```python
from build123d import *

# Parameters (mm, degrees)
F0_R     = 12.7
F1_DEPTH = 25.4
F2_R     = 12.7
F3_DEPTH = 50.8
F4_R     = 12.7


with BuildPart() as f1:
    # F0 (on Front) → F1 (new body)
    with BuildSketch(Plane.XZ):
        with BuildLine():
            Line((60.317927, -4.766353), (-27.044199, 54.367976))
            ThreePointArc((-27.044199, 54.367976), (-53.188332, 55.770247), (-66.682073, 33.333647))
            Line((-66.682073, 33.333647), (-66.682073, -17.466353))
            Line((-66.682073, -17.466353), (60.317927, -17.466353))
            Line((60.317927, -17.466353), (60.317927, -4.766353))
        make_face()
        with Locations((-41.282073, 33.333647)):
            Circle(F0_R, mode=Mode.SUBTRACT)
    extrude(amount=F1_DEPTH)

    # F2 (on Front) → F3 (join)
    with BuildSketch(Plane.XZ):
        with BuildLine():
            Line((-15.862083, -4.67199), (-15.862083, 33.193771))
            ThreePointArc((-15.862083, 33.193771), (-41.262083, 58.593771), (-66.662083, 33.193771))
            ThreePointArc((-66.662083, 33.193771), (-66.662036, 33.145056), (-66.661896, 33.096341))
            Line((-66.661896, 33.096341), (-66.58946, -4.67199))
            Line((-66.58946, -4.67199), (-66.58946, -17.566571))
            Line((-66.58946, -17.566571), (60.406737, -17.566571))
            Line((60.406737, -17.566571), (60.406737, -4.67199))
            Line((60.406737, -4.67199), (-15.862083, -4.67199))
        make_face()
        with Locations((-41.262083, 33.193771)):
            Circle(F2_R, mode=Mode.SUBTRACT)
    extrude(amount=F3_DEPTH)

    # F4
    f4_edges = [f1.edges().sort_by_distance(p)[0] for p in [
        (60.406737, -50.8, -11.11928),
    ]]
    fillet(f4_edges, radius=F4_R)


solid = f1.part
```
Geometry: final body of the model. Coordinates: model frame, mm. A direction names the side the tool comes from. Coordinates: 2 decimals unless noted, no trailing zeros. Loops run counter-clockwise (first coordinate to the right, second up) from the corner with the lowest first, then second, coordinate; pieces in that order, holes last. Notation, with made-up numbers: M 41,30.25 L 98,30.25 A21 ccw 98,45.25 Z; hole C -18,49.5 d11. An arc over 180 degrees is marked long. Put each result on its own line as item: value.
(1) Material intervals for probe 1 along X at (y, z) = (-31, -5); probe 2 along X at (y, z) = (-6, 39); probe 3 along Z at (x, y) = (-27, -17), sorted ascending.
Answer sheet:
probe 1: x = -66.59 to 60.41
probe 2: x = -66.04 to -52.56, -29.97 to -4.34
probe 3: z = -17.57 to 54.34
(2) Cut plane A-A on y = -34. Return the cut outline in (x, z).
Answer sheet:
outline: M -66.66,33.1 L -66.59,-4.67 L -66.59,-17.57 L 60.41,-17.57 L 60.41,-4.67 L -15.86,-4.67 L -15.86,33.19 A25.4 ccw -66.66,33.19 A25.52 ccw Z; hole C -41.26,33.19 d25.4
(3) Cut plane D-D on z = 9.5. Return the cut outline in (x, y).
Answer sheet:
outline: M -66.68,-25.4 L -66.62,-25.4 L -66.62,-50.8 L -15.86,-50.8 L -15.86,-25.4 L 39.24,-25.4 L 39.24,0 L -66.68,0 Z
(4) Draft query along X for faces 1 (the face through (-39.761, -12.522, 20.725)), 2 (the face through (-52.847, -12.522, 55.948)), 3 (the face through (-15.862, -38, 14)). Return one class per face: pulls with the +X half, pulls with the -X half, needs draft (parallel to the pull), parting line crosses it, or undercut.
Answer sheet:
face 1: undercut
face 2: parting line crosses it
face 3: pulls with the +X half
(5) Cut plane C-C on z = 40.5. Return the cut outline in (x, y).
Answer sheet:
outline: M -65.65,-25.4 L -65.59,-25.4 L -65.59,-50.8 L -51.65,-50.8 L -51.65,0 L -65.65,0 Z; M -30.87,-50.8 L -16.94,-50.8 L -16.94,-25.4 L -6.56,-25.4 L -6.56,0 L -30.87,0 Z
(6) Cut plane B-B on x = -45.5. Return the cut outline in (y, z).
Answer sheet:
outline: M -50.8,-17.57 L 0,-17.57 L 0,21.35 L -25.4,21.35 L -25.4,21.22 L -50.8,21.22 Z; M -50.8,45.17 L 0,45.17 L 0,58.38 L -25.4,58.38 L -25.4,58.24 L -50.8,58.24 Z
(7) First-contact query: pin 1 (12 mm diameter, centred on x = 38.5, z = 7.5, fed in from -Y); pin 2 (1.5 mm diameter, centred on x = 17.5, y = -21.5, fed in from +Z); pin 3 (3 mm diameter, centred on y = -22.5, z = 21, fed in from +X). Flat tips, straight axial feed; report the tip coordinate or a pass-through.
Answer sheet:
pin 1: stops at y = -25.4
pin 2: stops at z = 24.72
pin 3: stops at x = 24.47
(8) Access query for faces 4 (the face through (-40.704, -37.922, 58.588)), 5 (the face through (56.588, -47.178, -11.029)), 6 (the face through (-18, 0, 13)), 7 (the face through (23, -36, -4.672)), 8 (the face through (-42.915, -30.689, 45.786)). Directions: +Z, -Z, +X, -X, +Y, -Y. A direction counts if a zero-diameter tool reaches every point of the face in a straight line with its end or side. Return the directions, or none.
Answer sheet:
face 4: +Z, -Y
face 5: +Z, -Z, +X, -Y
face 6: +Z, -Z, +X, -X, +Y
face 7: +Z, +X, -Y
face 8: -Y
